The model under review builds one solid part; all positions refer to its coordinate system, in mm. Face numbers are marked on the shaded views. A direction names the side the tool comes from. Give positions to 0.01 mm unless a question says otherwise; leave off trailing zeros. Order: outer loops, then holes, each group sorted by start corner. A loop starts at its lowest first (then second) coordinate and runs counter-clockwise, first axis right, second up. Notation, with made-up numbers: (46, 65.25) - (71, 65.25) arc R33 cw to (71, 104.25) - close; hole circle Ø8 at (57.5, -23). An arc over 180 degrees is marked (long way). Write item = value, one per line. Start each with the question number.
1. We need section C-C, the plane x = 0. Give the boundary of the cut face in (y, z), and give its area (3 significant figures).
2. We need section D-D, the plane y = 2.5. Give the boundary of the cut face in (x, z).
3. Mouldability with a two-part tool opening along X and no side actions: class the marked faces 1, 2 and 3 as pulls with the +X half, pulls with the -X half, needs draft (parallel to the pull), parting line crosses it, or undercut.
4. Machinability: for the marked faces 4, 5, 6 and 7, which of the approach directions +Z, -Z, +X, -X, +Y, -Y give a long, thin tool a straight path to every point of the face, cutting with its end or side? Answer none if there is none.
5. We need section B-B, the plane y = 13.5. Give the boundary of the cut face in (x, z), and give its area (3 significant figures).
6. Wall thickness on probe 1 along X at (y, z) = (8.75, -5); probe 2 along X at (y, z) = (2.9, 0); probe 3 along X at (y, z) = (6.5, -4.25): over which ranges is each line inside the solid? List them lowest first.
7. For P1, Ø3, axis at x = -46.07, z = 5, coming from the +Y side; P2, Ø2, axis at x = 34.5, z = -5, coming from the -Y side; P3, Ø1.6, axis at x = 37.5, y = 21, coming from the -Z side; P4, Ø11.5, axis at x = 23.5, y = 6, coming from the -Z side, all flat-tipped, find the tip position at first contact; note any pin that passes through.
8. We need section A-A, the plane z = 0. Give the boundary of the cut face in (x, y), and give its area (3 significant figures).
from build123d import *

# Parameters (mm, degrees)
SKETCH1_W               = 88
SKETCH1_H               = 20
BOSS_EXTRUDE1_DEPTH     = 48
SKETCH2_R               = 4.25
CUT_EXTRUDE1_DEPTH      = 21
SKETCH7_R               = 12.5
BOSS_EXTRUDE2_DEPTH     = 48
SKETCH4_R               = 8.2
CUT_EXTRUDE3_DEPTH      = 49
FILLET2_R               = 10
SKETCH9_W               = 27
SKETCH9_H               = 25
CUT_EXTRUDE4_DEPTH      = 89
SKETCH10_W              = 63.73864418
SKETCH10_H              = 20
CUT_EXTRUDE5_DEPTH      = 13.5
CUT_EXTRUDE5_DEPTH_BACK = 13.5
FILLET3_R               = 5
SKETCH11_W              = 20
SKETCH11_H              = 23
BOSS_EXTRUDE3_DEPTH     = 6
SKETCH12_R              = 1.6
CUT_EXTRUDE6_DEPTH      = 24
FILLET5_R               = 5
BOSS_EXTRUDE4_DEPTH     = 4


with BuildPart() as part:
    # Sketch1 → Boss-Extrude1 (new body)
    with BuildSketch(Plane(origin=(0, 0, 0), x_dir=(1, 0, 0), z_dir=(0, 1, 0))):
        Rectangle(SKETCH1_W, SKETCH1_H)
    extrude(amount=BOSS_EXTRUDE1_DEPTH)

    # Sketch2 → Cut-Extrude1 (cut, through all)
    with BuildSketch(Plane.XY.offset(10)):
        with Locations((-38, 24)):
            Circle(SKETCH2_R)
        with Locations((38, 24)):
            Circle(SKETCH2_R)
    extrude(amount=-CUT_EXTRUDE1_DEPTH, mode=Mode.SUBTRACT)

    # Sketch7 → Boss-Extrude2 (add)
    with BuildSketch(Plane(origin=(0, 48, 0), x_dir=(1, 0, 0), z_dir=(0, 1, 0))):
        Circle(SKETCH7_R)
    extrude(amount=-BOSS_EXTRUDE2_DEPTH)

    # Sketch4 → Cut-Extrude3 (cut, through all)
    with BuildSketch(Plane(origin=(0, 48, 0), x_dir=(1, 0, 0), z_dir=(0, 1, 0))):
        Circle(SKETCH4_R)
    extrude(amount=-CUT_EXTRUDE3_DEPTH, mode=Mode.SUBTRACT)

    # Fillet2
    fillet2_edges = [part.edges().sort_by_distance(p)[0] for p in [
        (7.5, 24, -10),
        (7.5, 24, 10),
        (-7.5, 24, -10),
        (-7.5, 24, 10),
    ]]
    fillet(fillet2_edges, radius=FILLET2_R)

    # Sketch9 → Cut-Extrude4 (cut, through all)
    with BuildSketch(Plane.ZY.offset(44)):
        with Locations((0, 35.5)):
            Rectangle(SKETCH9_W, SKETCH9_H)
    extrude(amount=-CUT_EXTRUDE4_DEPTH, mode=Mode.SUBTRACT)

    # Sketch10 → Cut-Extrude5 (cut, two sides)
    with BuildSketch(Plane.XY) as cut_extrude5_sk:
        with Locations((0, 15)):
            Rectangle(SKETCH10_W, SKETCH10_H)
    extrude(amount=CUT_EXTRUDE5_DEPTH, mode=Mode.SUBTRACT)
    extrude(cut_extrude5_sk.sketch, amount=-CUT_EXTRUDE5_DEPTH_BACK, mode=Mode.SUBTRACT)

    # Fillet3
    fillet3_edges = [part.edges().sort_by_distance(p)[0] for p in [
        (31.86932209, 5, 0),
        (-31.86932209, 5, 0),
    ]]
    fillet(fillet3_edges, radius=FILLET3_R)

    # Sketch11 → Boss-Extrude3 (add)
    with BuildSketch(Plane(origin=(44, 0, 0), x_dir=(0, 0, -1), z_dir=(1, 0, 0))):
        with Locations((0, 11.5)):
            Rectangle(SKETCH11_W, SKETCH11_H)
    boss_extrude3 = extrude(amount=BOSS_EXTRUDE3_DEPTH)

    # Sketch12 → Cut-Extrude6 (cut, through all)
    with BuildSketch(Plane(origin=(0, 23, 0), x_dir=(1, 0, 0), z_dir=(0, 1, 0))):
        with Locations((46.065338955, 5)):
            Circle(SKETCH12_R)
        with Locations((46.065338955, -5)):
            Circle(SKETCH12_R)
    cut_extrude6 = extrude(amount=-CUT_EXTRUDE6_DEPTH, mode=Mode.SUBTRACT)

    # Mirror1: Boss-Extrude3, Cut-Extrude6 across plane
    add(boss_extrude3.mirror(Plane(origin=(0, 0, 0), x_dir=(0, 0, 1), z_dir=(1, 0, 0))))
    add(cut_extrude6.mirror(Plane(origin=(0, 0, 0), x_dir=(0, 0, 1), z_dir=(1, 0, 0))), mode=Mode.SUBTRACT)

    # Fillet5
    fillet5_edges = [part.edges().sort_by_distance(p)[0] for p in [
        (50, 11.5, -10),
        (50, 11.5, 10),
        (-50, 11.5, 10),
        (-50, 11.5, -10),
    ]]
    fillet(fillet5_edges, radius=FILLET5_R)

    # Sketch13 → Boss-Extrude4 (add)
    with BuildSketch(Plane.XY.offset(10)):
        with BuildLine():
            Line((-42.13067791, 23), (-33.86932209, 23))
            ThreePointArc((-33.86932209, 23), (-38, 19.75), (-42.13067791, 23))
        make_face()
        with BuildLine():
            Line((33.86932209, 23), (42.13067791, 23))
            ThreePointArc((42.13067791, 23), (38, 19.75), (33.86932209, 23))
        make_face()
    extrude(amount=-BOSS_EXTRUDE4_DEPTH)


solid = part.part
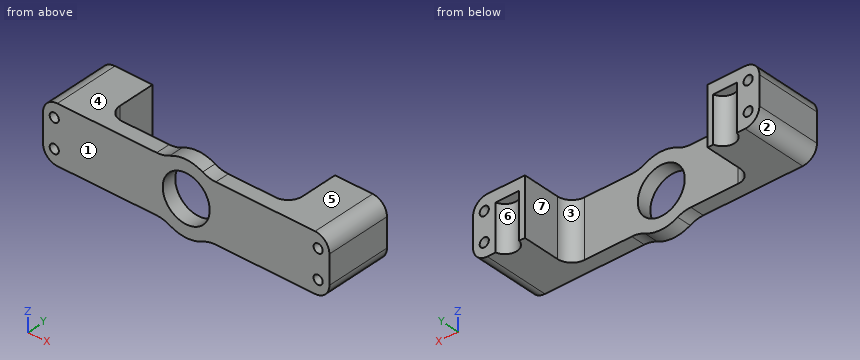
Model answer:
q1.outline = (0, -12.5) - (5, -12.5) - (5, -8.2) - (0, -8.2) - close; (0, 8.2) - (5, 8.2) - (5, 12.5) - (0, 12.5) - close
q1.area = 43.0 mm2
q2.outline = (-50, -5) arc R5 ccw to (-45, -10) - (-10.31, -10) arc R10 cw to (-5.73, -11.11) arc R12.5 ccw to (5.73, -11.11) arc R10 cw to (10.31, -10) - (45, -10) arc R5 ccw to (50, -5) - (50, 5) arc R5 ccw to (45, 10) - (10.31, 10) arc R10 cw to (5.73, 11.11) arc R12.5 ccw to (-5.73, 11.11) arc R10 cw to (-10.31, 10) - (-45, 10) arc R5 ccw to (-50, 5) - close; hole circle Ø3.2 at (-46.07, -5); hole circle Ø3.2 at (-46.07, 5); hole circle Ø16.4 at (0, 0); hole circle Ø3.2 at (46.07, -5); hole circle Ø3.2 at (46.07, 5)
q3.face_1 = needs draft
q3.face_2 = pulls with the -X half
q3.face_3 = undercut
q4.face_4 = +Z, -X, +Y, -Y
q4.face_5 = +Z, +X, +Y, -Y
q4.face_6 = -Z, +Y
q4.face_7 = +Z, -Z, +Y
q5.outline = (-50, -5) arc R5 ccw to (-45, -10) - (-31.87, -10) - (-31.87, 10) - (-45, 10) arc R5 ccw to (-50, 5) - close; (31.87, -10) - (45, -10) arc R5 ccw to (50, -5) - (50, 5) arc R5 ccw to (45, 10) - (31.87, 10) - close; hole circle Ø3.2 at (-46.07, -5); hole circle Ø3.2 at (-46.07, 5); hole circle Ø3.2 at (46.07, -5); hole circle Ø3.2 at (46.07, 5)
q5.area = 672 mm2
q6.probe_1 = -50 to -47.67, -44.47 to -31.71, 31.71 to 44.47, 47.67 to 50
q6.probe_2 = -50 to -8.2, 8.2 to 50
q6.probe_3 = -50 to -47.48, -44.65 to -30.44, 30.44 to 44.65, 47.48 to 50
q7.P1 = through
q7.P2 = 0
q7.P3 = 6
q7.P4 = -10
q8.outline = (-50, 0) - (-8.2, 0) - (-8.2, 5) - (-26.87, 5) arc R5 cw to (-31.87, 10) - (-31.87, 23) - (-33.87, 23) arc R4.25 cw to (-42.13, 23) - (-50, 23) - close; (8.2, 0) - (50, 0) - (50, 23) - (42.13, 23) arc R4.25 cw to (33.87, 23) - (31.87, 23) - (31.87, 10) arc R5 cw to (26.87, 5) - (8.2, 5) - close
q8.area = 1,040 mm2
